Can you work these out from the drawing? Everything is in mm from the part's minimum corner. A direction names the side the tool comes from. Round coordinates to 2 decimals unless told otherwise and drop trailing zeros. Loops run counter-clockwise (first coordinate to the right, second up) from the corner with the lowest first, then second, coordinate; pieces in that order, holes last. Notation, with made-up numbers: M 42,9 L 69,9 A11 cw 69,30 Z; hole C 37,28 d10. An arc over 180 degrees is marked long. Return JSON: item names as keys, results as strings. Group by question number.
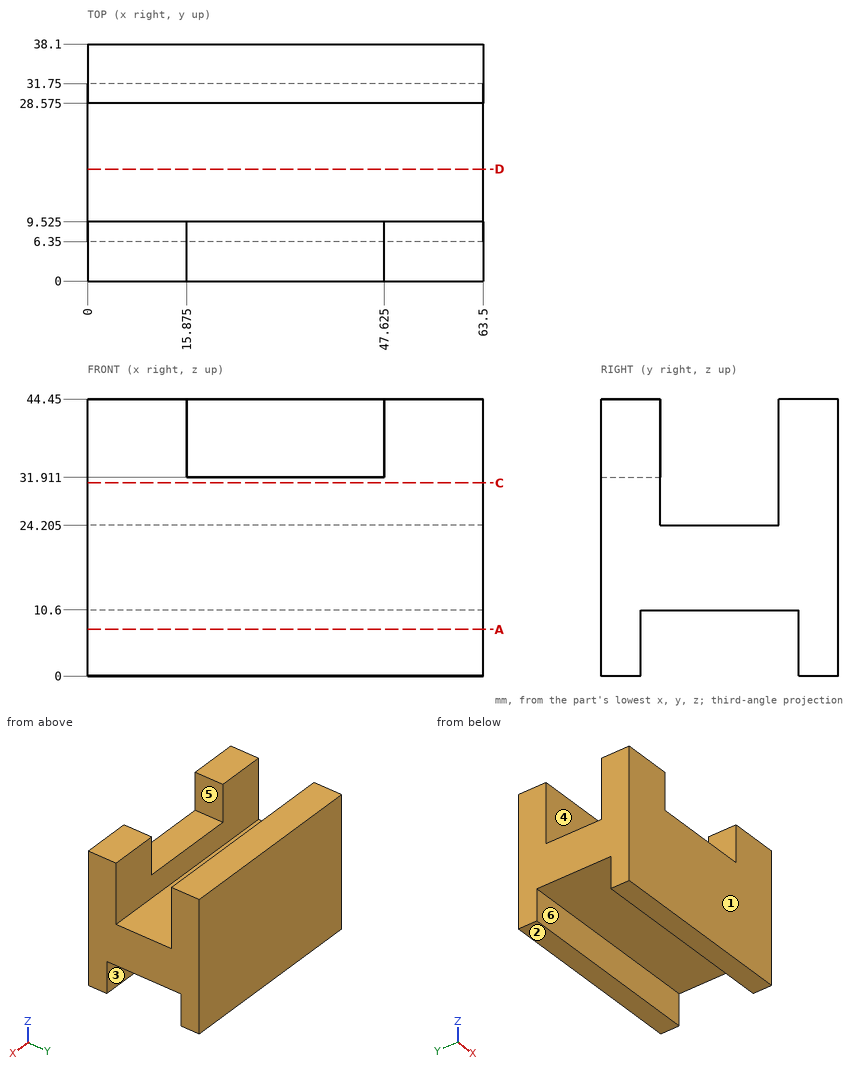
1. If we section it at A-A, the plane z = 7.5: Please give me the cut outline in (x, y).
2. I need wall thicknesses on probe 1 along Y at (x, z) = (41, 3); probe 2 along Y at (x, z) = (6.5, 34) (1 decimal); probe 3 along Z at (x, y) = (15, 9). Which ranges of each line are inside material? Lowest first, please.
3. We'd pull the mould along Y, two halves only. Please class the marked faces 1, 2 and 3: +Y half, -Y half, draft (parallel to the pull), parting line (faces both ways), or undercut.
4. If we section it at C-C, the plane z = 31: Please give me the cut outline in (x, y) (1 decimal).
5. On a 3-axis mill with a long thin cutter (end or side, diameter ignored), from which of +Z, -Z, +X, -X, +Y, -Y can I reach the whole of each face in a straight line? I mean the marked faces 4, 5 and 6. Say none if no direction works.
6. If we section it at D-D, the plane y = 18: Please give me the cut outline in (x, z) (1 decimal), then the cut area to 3 significant figures.
7. I'm going to push flat-ended pins straight in: pin 1 Ø8 at (x, y) = (39, 18) entering from +Z (3 decimals); pin 2 Ø12 at (x, y) = (14.5, 17) entering from -Z; pin 3 Ø5 at (x, y) = (30, 3) entering from +Z. Where does each tip first touch, or does it pass through?
Geometry results:
{
 "1": {"outline": "M 0,0 L 63.5,0 L 63.5,6.35 L 0,6.35 Z; M 0,31.75 L 63.5,31.75 L 63.5,38.1 L 0,38.1 Z"},
 "2": {"probe 1": "0 to 6.35, 31.75 to 38.1", "probe 2": "0 to 9.5, 28.6 to 38.1", "probe 3": "10.6 to 44.45"},
 "3": {"face 1": "-Y half", "face 2": "draft", "face 3": "undercut"},
 "4": {"outline": "M 0,0 L 63.5,0 L 63.5,9.5 L 0,9.5 Z; M 0,28.6 L 63.5,28.6 L 63.5,38.1 L 0,38.1 Z"},
 "5": {"face 4": "+Z, +X, -X", "face 5": "+Z, -Y", "face 6": "-Z, +X, -X"},
 "6": {"outline": "M 0,10.6 L 63.5,10.6 L 63.5,24.2 L 0,24.2 Z", "area": "864 mm^2"},
 "7": {"pin 1": "z = 24.205", "pin 2": "z = 10.6", "pin 3": "z = 31.91"}
}
